Can you work these out from the model? Positions are in its coordinate system, mm. Face numbers are marked on the shaded views. A direction names the side the tool comes from. Coordinates: 2 decimals unless noted, no trailing zeros. Loops run counter-clockwise (first coordinate to the right, second up) from the corner with the lowest first, then second, coordinate; pieces in that order, holes last.
Autodesk Inventor part; units mm, degrees
ref_plane "YZ Plane" through (0, 0, 0) normal (1, 0, 0) x (0, 1, 0)
ref_plane "XZ Plane" through (0, 0, 0) normal (0, 1, 0) x (-1, 0, 0)
ref_plane "XY Plane" through (0, 0, 0) normal (0, 0, 1) x (1, 0, 0)
sketch "Sketch5" plane through (0, 0, 0) normal (0, 1, 0) x (-1, 0, 0)
  line L0 (-272.8857, 16.2919) -> (-285.5857, 16.2919)
  line L1 (-285.5857, 16.2919) -> (-285.5857, 21.0544)
  line L2 (-285.5857, 21.0544) -> (-280.6644, 21.0544)
  line L3 (-280.6644, 26.3249) -> (-285.5857, 26.3249)
  line L4 (-280.6644, 21.0544) -> (-280.6644, 26.3249)
  line L5 (-280.6644, 31.0874) -> (-285.5857, 31.0874)
  line L6 (-285.5857, 26.3249) -> (-285.5857, 31.0874)
  line L7 (-280.6644, 31.0874) -> (-280.6644, 36.3579)
  line L8 (-285.5857, 36.3579) -> (-285.5857, 41.1204)
  line L9 (-285.5857, 41.1204) -> (-266.3769, 41.1204)
  line L10 (-272.8857, 9.9419) -> (-272.8857, 16.2919)
  line L11 (-266.3769, -18.3156) -> (-266.3769, 41.1204)
  line L12 (-291.7769, 9.9419) -> (-272.8857, 9.9419)
  line L13 (-282.7599, -18.3156) -> (-266.3769, -18.3156)
  line L14 (-291.7769, 6.7669) -> (-282.7599, -18.3156)
  line L15 (-291.7769, 6.7669) -> (-291.7769, 9.9419)
  line L16 (-280.6644, 36.3579) -> (-285.5857, 36.3579)
  line L17 (-342.5769, -58.268) -> (-342.5769, 69.8263)
  line L18 (-266.3769, -0.8164) -> (-269.5519, -0.8164)
  line L19 (-269.5519, -0.8164) -> (-269.5519, 2.3586)
  line L20 (-269.5519, 2.3586) -> (-266.3769, 2.3586)
  point P0 (0, 0)
  dimension "d34" = 3.175
  dimension "d35" = 9.017
  dimension "d36" = 50.8
  dimension "d37" = 76.2
  dimension "d39" = 61.9125
  dimension "d40" = 6.35
  dimension "d41" = 56.9913
  dimension "d42" = 12.7
  dimension "d43" = 3.175
  dimension "d44" = 3.175
  dimension "d45" = 17.4992
  dimension "d46" = 28.2575
  dimension "d47" = 4.7625
revolve "Revolution2" add sketch "Sketch5" angle 360 about axis through (342.5769, 0, -58.268) along (0, 0, 1) contours L0 L1 L2 L4 L3 L6 L5 L7 L16 L8 L9 L11 L20 L19 L18 L13 L14 L15 L12 L10
equation "\"d41\" = 0.5 * WashChamberOD - SealedSurfaceOffset"
equation "\"d47\" = StaticORingThickness"
equation "\"MachineMaxHeight\" = 539.75"
equation "\"MachineMaxWidth\" = 215.9"
equation "\"MachineMaxLength\" = 266.7"
equation "\"MachineFluidCapacity\" = 25.4"
equation "\"MaxCompressiveCapacity\" = 20320"
equation "\"WashChamberID\" = 101.6"
equation "\"WashChamberOD\" = 114.3"
equation "\"ConduitThickness\" = 152.4"
equation "\"StaticORingThickness\" = 4.7625"
equation "\"SealedSurfaceOffset\" = 0.15875"
properties part number "WashChamberConduit"
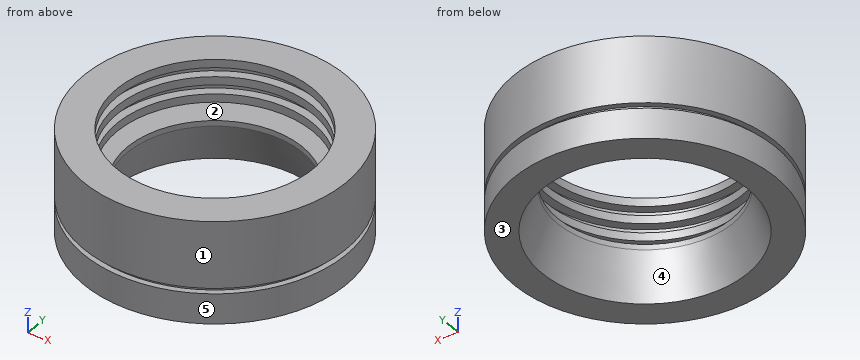
(1) If I drill on probe 1 along X at (y, z) = (0, 34.5); probe 2 along X at (y, z) = (0, 19.9); probe 3 along Z at (x, y) = (278, 19), over which ranges is the centre line in solid material (lowest first)?
Check values:
probe 1: x = 266.38 to 280.66, 404.49 to 418.78
probe 2: x = 266.38 to 285.59, 399.57 to 418.78
probe 3: z = -18.32 to 9.94, 16.29 to 41.12
(2) I'm going to push flat-ended pins straight in: pin 1 (1 mm diameter, centred on x = 370.5, z = 34, fed in from +Y); pin 2 (12 mm diameter, centred on y = 39.5, z = 14, fed in from -X); pin 3 (8 mm diameter, centred on y = -55.5, z = 25.5, fed in from -X). Where does each tip first touch, or does it pass through?
Check values:
pin 1: stops at y = 71.09
pin 2: stops at x = 274.14
pin 3: stops at x = 286.41
(3) If we mould it in two halves opening along X, with no side actions, what happens to the marked faces 3, 4 and 5? For each: released by +X, released by -X, zero draft, split by the parting line, or undercut.
Check values:
face 3: zero draft
face 4: undercut
face 5: split by the parting line
(4) I want a section at A-A on x = 407.5. Write out the boundary of the cut face in (y, z), then the cut area to 3 significant figures.
Check values:
outline: (-39.89, -18.32) - (39.89, -18.32) - (39.89, -0.82) - (33.43, -0.82) - (33.43, 2.36) - (39.89, 2.36) - (39.89, 41.12) - (-39.89, 41.12) - (-39.89, 2.36) - (-33.43, 2.36) - (-33.43, -0.82) - (-39.89, -0.82) - close; hole (-25.33, 9.94) - (25.33, 9.94) - (25.33, 16.29) - (-25.33, 16.29) - close
area: 4,380 mm2
(5) Which directions (+Z, -Z, +X, -X, +Y, -Y) give clear straight access to the entire face, cutting with the end or side of a thin tool? Please do the marked faces 1 and 2.
Check values:
face 1: +Z, -Z
face 2: none
